Can you work these out from the drawing? Everything is in mm from the part's minimum corner. A direction names the side the tool comes from. Give positions to 0.01 mm unless a question says otherwise; leave off trailing zeros. Loops run counter-clockwise (first coordinate to the right, second up) from the corner with the lowest first, then second, coordinate; pieces in that order, holes last. Notation, with made-up numbers: (88.5, 65) -> (106.5, 65) arc R26 ccw to (106.5, 96) -> close; hole circle Ø3 at (62.25, 25). An arc over 180 degrees is marked (long way). Write item = value, one per line. Start each with the question number.
1) I'm going to push flat-ended pins straight in: pin 1 Ø5 at (y, z) = (34.925, 98.425) entering from -X; pin 2 Ø1.5 at (x, y) = (8, 17.5) entering from -Z; pin 3 Ø6 at (y, z) = (28, 41.5) entering from -X; pin 4 Ø2 at (x, z) = (5.5, 63.5) entering from -Y. Where does each tip first touch, or does it pass through?
2) I want a section at C-C (y = 37). List the corners of the cut face in (x, z) for me.
3) I need wall thicknesses on probe 1 along Y at (x, z) = (16, 15) (1 decimal); probe 2 along Z at (x, y) = (8.5, 20) (1 decimal); probe 3 along Y at (x, z) = (3, 64) (1 decimal). Which ranges of each line are inside material? Lowest first, please. Write a range as from..to.
4) If we mould it in two halves opening along X, with no side actions, what happens to the marked faces 1, 2 and 3? For each: +X half, -X half, draft (parallel to the pull), parting line (faces both ways), or undercut.
5) On a 3-axis mill with a long thin cutter (end or side, diameter ignored), from which of +Z, -Z, +X, -X, +Y, -Y can I reach the whole of each face in a straight line? I mean the marked faces 4 and 5. Say none if no direction works.
6) I want a section at B-B (x = 20). List the corners of the cut face in (y, z) for me (1 decimal), and give its area (3 significant figures).
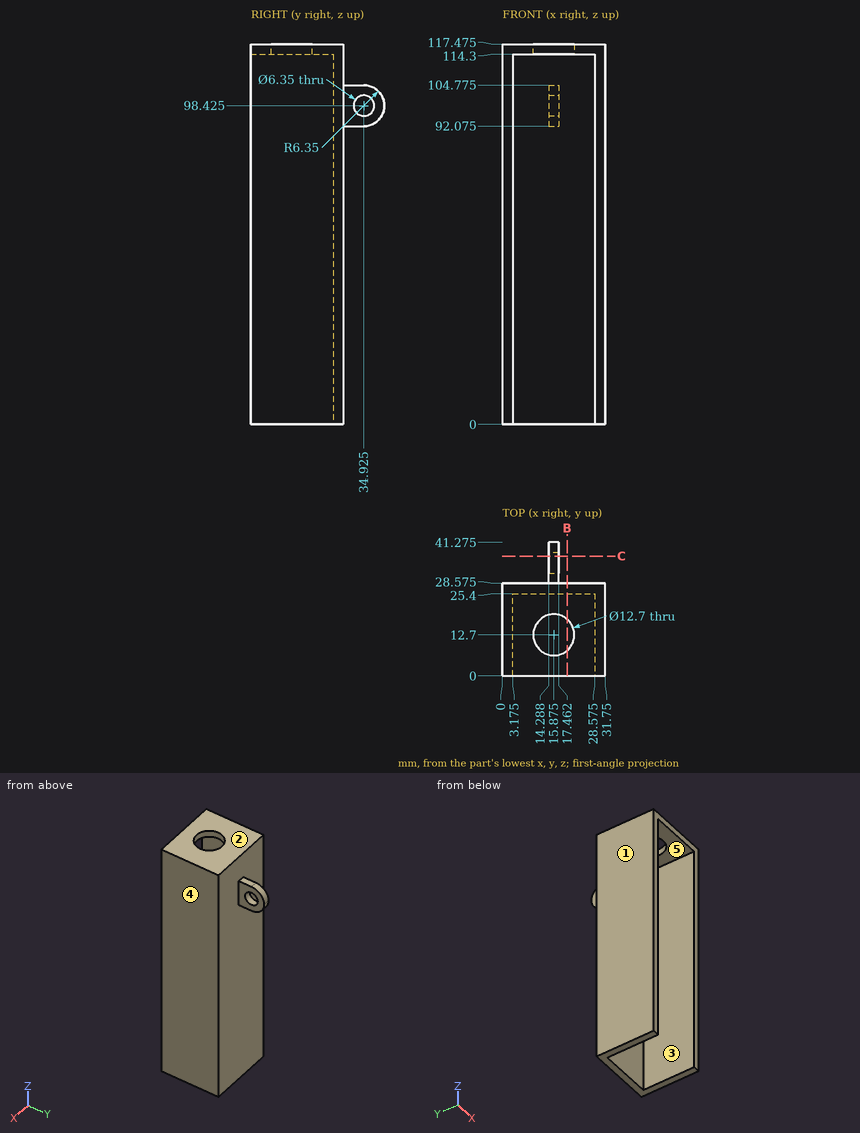
Answer list:
q1.pin_1 = through
q1.pin_2 = 114.3
q1.pin_3 = 0
q1.pin_4 = 25.4
q2.outline = (14.29, 92.42) -> (17.46, 92.42) -> (17.46, 96.02) -> (14.29, 96.02) -> close; (14.29, 100.83) -> (17.46, 100.83) -> (17.46, 104.43) -> (14.29, 104.43) -> close
q3.probe_1 = 25.4..28.6
q3.probe_2 = 114.3..117.5
q3.probe_3 = 0..28.6
q4.face_1 = -X half
q4.face_2 = draft
q4.face_3 = undercut
q5.face_4 = +Z, -Z, +X, +Y, -Y
q5.face_5 = -Z, -Y
q6.outline = (0, 114.3) -> (7.9, 114.3) -> (7.9, 117.5) -> (0, 117.5) -> close; (17.5, 114.3) -> (25.4, 114.3) -> (25.4, 0) -> (28.6, 0) -> (28.6, 117.5) -> (17.5, 117.5) -> close
q6.area = 423 mm^2
